The model under review builds one solid part; all positions refer to its coordinate system, in mm. Face numbers are marked on the shaded views. A direction names the side the tool comes from. Give positions to 0.01 mm unless a question says otherwise; leave off trailing zeros. Order: outer loops, then holes, each group sorted by start corner. A loop starts at its lowest first (then second) coordinate and runs counter-clockwise, first axis right, second up.
```python
from build123d import *

# Parameters (mm, degrees)
ESQUISSE2_W             = 20
ESQUISSE2_H             = 40
BOSS_EXTRU_2_DEPTH      = 20
BOSS_EXTRU_3_DEPTH      = 10
ESQUISSE6_W             = 50
ESQUISSE6_H             = 20
ESQUISSE6_R             = 2.5
BOSS_EXTRU_4_DEPTH      = 5
ESQUISSE8_R             = 1.5
ENL_V_MAT_EXTRU_1_DEPTH = 40
CONG_2_R                = 10
CONG_3_R                = 10
CHANFREIN2_SIZE         = 10
CHANFREIN2_SIZE2        = 9.656887748


with BuildPart() as part:
    # Esquisse2 → Boss.-Extru.2 (new body)
    with BuildSketch(Plane.XY):
        with Locations((10, -20)):
            Rectangle(ESQUISSE2_W, ESQUISSE2_H)
    extrude(amount=BOSS_EXTRU_2_DEPTH)

    # Esquisse3 → Boss.-Extru.3 (add)
    with BuildSketch(Plane.XY.offset(20)):
        with BuildLine():
            Line((0, 15), (0, 0))
            Line((0, 0), (20, 0))
            Line((20, 0), (20, 7.210541204))
            Line((20, 7.210541204), (14.490680751, 7.210541204))
            ThreePointArc((14.490680751, 7.210541204), (5.50498976, 7.288144059), (14.443549392, 8.210541204))
            Line((14.443549392, 8.210541204), (20, 8.210541204))
            Line((20, 8.210541204), (20, 15))
            Line((20, 15), (0, 15))
        make_face()
    extrude(amount=-BOSS_EXTRU_3_DEPTH)

    # Esquisse6 → Boss.-Extru.4 (add)
    with BuildSketch(Plane.XZ.offset(40)):
        with Locations((10, 10)):
            Rectangle(ESQUISSE6_W, ESQUISSE6_H)
        with Locations(Location((-7.5, 10, 0), (0, 0, 270))):
            Circle(ESQUISSE6_R, mode=Mode.SUBTRACT)
        with Locations(Location((27.5, 10, 0), (0, 0, 270))):
            Circle(ESQUISSE6_R, mode=Mode.SUBTRACT)
    extrude(amount=-BOSS_EXTRU_4_DEPTH)

    # Esquisse8 → Enlèv. mat.-Extru.1 (cut)
    with BuildSketch(Plane(origin=(0, 15, 0), x_dir=(1, 0, 0), z_dir=(0, 1, 0))):
        with Locations(Location((16.757752744, -15, 0), (0, 0, 270))):
            Circle(ESQUISSE8_R)
    extrude(amount=-ENL_V_MAT_EXTRU_1_DEPTH, mode=Mode.SUBTRACT)

    # Congé2
    cong_2_edges = [part.edges().sort_by_distance(p)[0] for p in [
        (0, 15, 15),
    ]]
    fillet(cong_2_edges, radius=CONG_2_R)

    # Congé3
    cong_3_edges = [part.edges().sort_by_distance(p)[0] for p in [
        (-15, -37.5, 0),
        (-15, -37.5, 20),
        (35, -37.5, 20),
        (35, -37.5, 0),
    ]]
    fillet(cong_3_edges, radius=CONG_3_R - 0.0001)  # a hair under: the kernel refuses the full size

    # Chanfrein2
    chanfrein2_edges = [part.edges().sort_by_distance(p)[0] for p in [
        (10, 0, 0),
    ]]
    chanfrein2_side = [part.faces().sort_by_distance(p)[0] for p in [
        (10, -21.029431142, 0),
    ]]
    chamfer(chanfrein2_edges, length=CHANFREIN2_SIZE, length2=CHANFREIN2_SIZE2, reference=chanfrein2_side[0])


solid = part.part
```
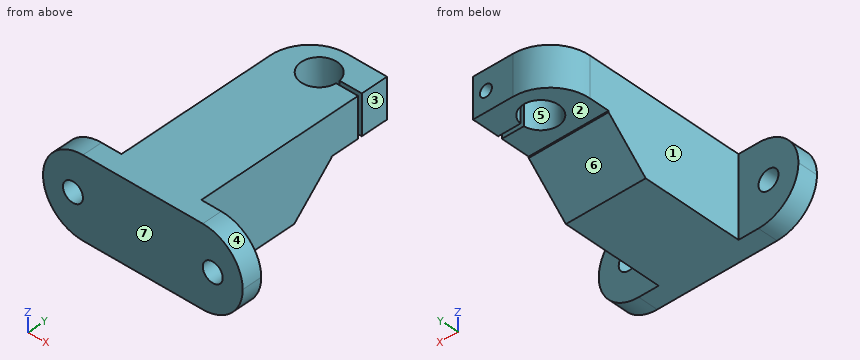
Item 1: Take a section at B-B (z = 14.5). Give the boundary of the cut face in (x, y).
Values found:
outline: (-13.93, -40) - (33.93, -40) - (33.93, -35) - (20, -35) - (20, 7.21) - (18.17, 7.21) - (18.17, -25) - (15.34, -25) - (15.34, 7.21) - (14.49, 7.21) arc R4.5 cw (long way) to (14.44, 8.21) - (15.34, 8.21) - (15.34, 15) - (10, 15) arc R10 ccw to (0, 5) - (0, -35) - (-13.93, -35) - close; (18.17, 8.21) - (20, 8.21) - (20, 15) - (18.17, 15) - close
Item 2: Take a section at A-A (x = 19). Give the boundary of the cut face in (y, z), and give its area (3 significant figures).
Values found:
outline: (-40, 0) - (-10, 0) - (0, 9.66) - (0, 10) - (7.21, 10) - (7.21, 20) - (-40, 20) - close; (8.21, 10) - (15, 10) - (15, 20) - (8.21, 20) - close
area: 892 mm2
Item 3: Draft analysis for pull direction Y (two halves, no side actions). For the marked faces 4, 5, 6 and 7, state which applies: released by +Y, released by -Y, zero draft, split by the parting line, or undercut.
Values found:
face 4: zero draft
face 5: undercut
face 6: released by +Y
face 7: released by -Y
Item 4: For the marked faces 1, 2 and 3, list the 3-axis set-ups (+Z, -Z, +X, -X, +Y, -Y) from which the entire face can be reached by the end or side of a thin tool; tool diameter is ignored.
Values found:
face 1: +Z, -Z, -X, +Y
face 2: -Z, +X, -X, +Y
face 3: +Z, -Z, +X, +Y
Item 5: For line 1 (Y direction, x = 10, z = 13); line 2 (Y direction, x = 15, z = 13.25); line 3 (X direction, y = -8.5, z = 15), list the stretches that pass through material, from the lowest coordinate up.
Values found:
line 1: y = -40 to 3, 12 to 15
line 2: y = -40 to 7.21, 8.21 to 15
line 3: x = 0 to 15.26, 18.26 to 20
Item 6: Take a section at C-C (z = 8.5). Give the boundary of the cut face in (x, y), and give its area (3 significant figures).
Values found:
outline: (-14.89, -40) - (-9.5, -40) - (-9.5, -35) - (-14.89, -35) - close; (-5.5, -40) - (25.5, -40) - (25.5, -35) - (20, -35) - (20, -1.2) - (0, -1.2) - (0, -35) - (-5.5, -35) - close; (29.5, -40) - (34.89, -40) - (34.89, -35) - (29.5, -35) - close
area: 885 mm2
Item 7: Take a section at D-D (y = -23). Give the boundary of the cut face in (x, z), and give its area (3 significant figures).
Values found:
outline: (0, 0) - (20, 0) - (20, 20) - (0, 20) - close; hole circle Ø3 at (16.76, 15)
area: 393 mm2
Item 8: Clearance check with flat-ended pins moving along their axes: pin 1 Ø8 at (x, z) = (-7.5, 10) entering from -Y; pin 2 Ø12 at (x, z) = (-10.5, 9.5) entering from +Y; pin 3 Ø12 at (y, z) = (-5.5, 14) entering from -X; pin 4 Ø6 at (x, z) = (0, 5) entering from +Y. State where each tip first meets the part, or that it passes through.
Values found:
pin 1: stops at y = -40
pin 2: stops at y = -35
pin 3: stops at x = 0
pin 4: stops at y = -1.72
